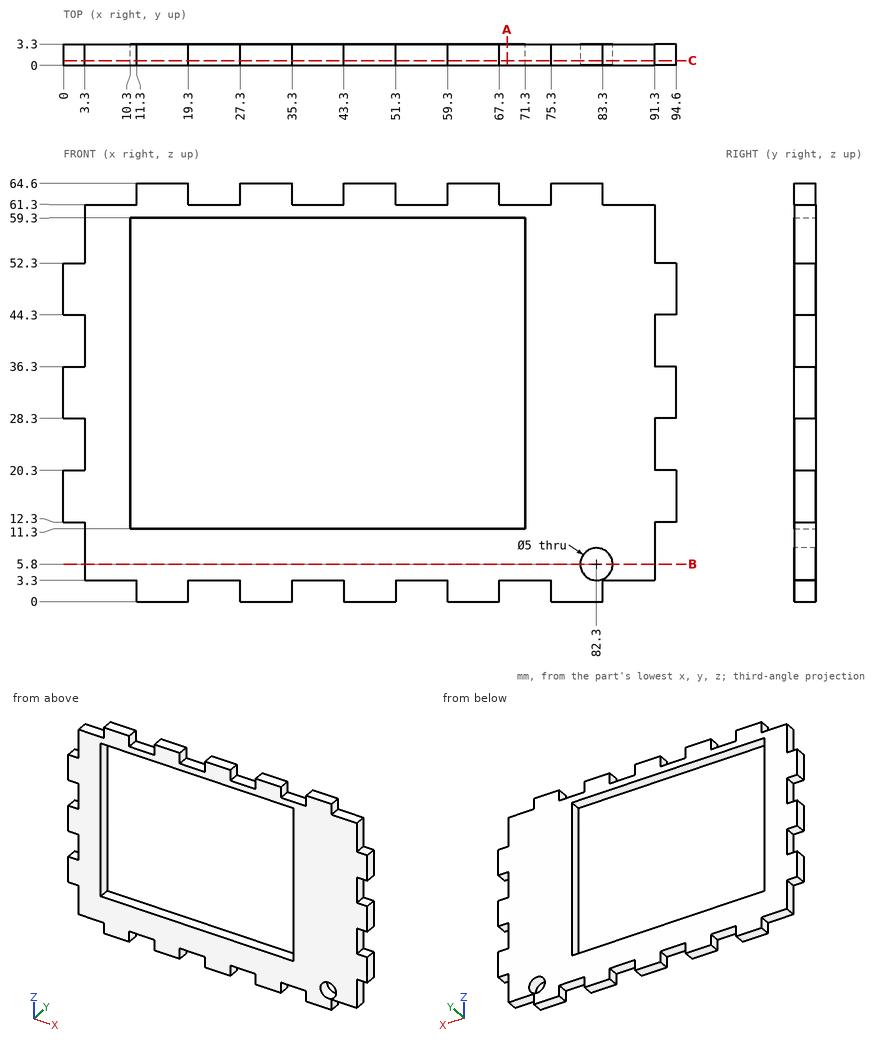
Verification items for this drawing (mm, ordinates from the low corner). Round coordinates to 2 decimals unless told otherwise and drop trailing zeros. Order: outer loops, then holes, each group sorted by start corner. A loop starts at its lowest first (then second) coordinate and runs counter-clockwise, first axis right, second up. Notation, with made-up numbers: M 55,21 L 112,21 A22 ccw 112,47 Z; hole C 7,73.5 d9. An arc over 180 degrees is marked long. Answer in a Markdown table with one row per item. Add a question column.
Item 1: Material ranges on L1, parallel to X at y = 1, z = 25; L2, parallel to X at y = 0.5, z = 52; L3, parallel to Z at x = 82.3, y = 1.95, recorded low to high. Write a range as [from, to].
Item 2: Sectioned sample at B-B, the plane z = 5.8. Enter the section's corners in (x, y), plus the area to 3 significant figures.
Item 3: Depth check by flat-ended pin: pin 1 Ø1.6 at (x, y) = (1, 1.5) entering from -Z; pin 2 Ø1.6 at (y, z) = (1.5, 42) entering from +X; pin 3 Ø1 at (x, y) = (39, 1.5) entering from -Z. Enter the tip coordinate at first touch or a pass-through.
Item 4: Sectioned sample at A-A, the plane x = 68.5. Enter the section's corners in (y, z).
Item 5: Sectioned sample at C-C, the plane y = 0.75. State how many separate pieces and enclosed holes the cut face has, plus the area to 3 significant figures.
Filled in:
| question | item | result |
|---|---|---|
| 1 | L1 | x = [3.3, 10.3], [71.3, 91.3] |
| 1 | L2 | x = [0, 10.3], [71.3, 94.6] |
| 1 | L3 | z = [0, 3.3], [8.3, 64.6] |
| 2 | outline | M 3.3,0 L 79.8,0 L 79.8,3.3 L 3.3,3.3 Z; M 84.8,0 L 91.3,0 L 91.3,3.3 L 84.8,3.3 Z |
| 2 | area | 274 mm² |
| 3 | pin 1 | stops at z = 12.3 |
| 3 | pin 2 | stops at x = 91.3 |
| 3 | pin 3 | stops at z = 3.3 |
| 4 | outline | M 0,3.3 L 3.3,3.3 L 3.3,11.3 L 0,11.3 Z; M 0,59.3 L 3.3,59.3 L 3.3,61.3 L 0,61.3 Z |
| 5 | separate pieces | 1 |
| 5 | enclosed holes | 2 |
| 5 | area | 2,580 mm² |
